Check sheet for the modelled part. Datum: model origin and axes. Units: mm. A direction names the side the tool comes from. Coordinates: 2 decimals unless noted, no trailing zeros. Loops run counter-clockwise (first coordinate to the right, second up) from the corner with the lowest first, then second, coordinate; pieces in that order, holes last. Notation, with made-up numbers: (-21, 3) - (0, 3) arc R8 cw to (0, 13) - close; hole circle Ø11 at (20.5, -30.75). An arc over 180 degrees is marked (long way). Write each question's results on one line, items separated by ' | '. Start each with the question number.
1. Gauge pin test, flat ends, axial feed: P1, Ø4, axis at y = 17, z = -13, coming from the -X side; P2, Ø4, axis at y = -12, z = 7.5, coming from the +X side; P3, Ø12, axis at x = -49.21, y = 4.19, coming from the -Z side; P4, Ø5, axis at y = -0.5, z = 9.5, coming from the +X side. Record the tip position at first contact, or that the pin passes through.
2. Cross-section at B-B (x = 48). Record the cut outline in (y, z), and give its area (3 significant figures).
3. Tool access check on faces 1 (the face through (-66, 3, 12.7)), 2 (the face through (-76.2, 3, 19)), 3 (the face through (-28.1, 12.878, -23.754)), 4 (the face through (-56, 6, 21.158)), 5 (the face through (42.78, 6.22, 23.25)). Record the directions out of +Z, -Z, +X, -X, +Y, -Y that give a thin tool (end or side, any length) a straight path to the whole face; none if there is none.
4. Thickness scan on line 1 (Y direction, x = 16.5, z = -19); line 2 (X direction, y = 8, z = 19.5); line 3 (Y direction, x = -45, z = 14.5). Record the ranges inside material, lowest first. Write a range as [from, to].
5. Cross-section at D-D (x = 13). Record the cut outline in (y, z).
6. Cross-section at C-C (z = 18). Record the cut outline in (x, y), and give its area (3 significant figures).
7. Draft check along Y on faces 6 (the face through (-1, -19.05, 6)), 7 (the face through (39.894, 0.792, 15.794)), 8 (the face through (65, 3, 12.7)). Enter one of: released by +Y, released by -Y, zero draft, split by the parting line, or undercut.
8. Cross-section at A-A (y = 16). Record the cut outline in (x, z).
```python
from build123d import *

# Parameters (mm, degrees)
BOSS_EXTRUDE1_DEPTH     = 25.4
BOSS_EXTRUDE2_DEPTH     = 6.604
SKETCH3_W               = 152.4
SKETCH3_H               = 50.8
BOSS_EXTRUDE3_DEPTH     = 12.446
SKETCH5_W               = 47.049242613
SKETCH5_H               = 38.1
CUT_EXTRUDE1_DEPTH      = 92.800885072
FILLET1_R               = 2.54
FILLET2_R               = 25.4
CUT_EXTRUDE2_DEPTH      = 8.4582
CUT_EXTRUDE2_DEPTH_BACK = 85.242269675
CUT_EXTRUDE2_START      = 12.7
SKETCH6_R               = 9.9187
SKETCH7_R               = 6.7437
CUT_EXTRUDE3_DEPTH      = 93.840002113


with BuildPart() as part:
    # Sketch1 → Boss-Extrude1 (new body)
    with BuildSketch(Plane(origin=(0, 0, 0), x_dir=(1, 0, 0), z_dir=(0, 1, 0))):
        with BuildLine():
            Line((76.2, -25.4), (76.2, 25.4))
            Line((76.2, 25.4), (29.150757387, 25.4))
            ThreePointArc((29.150757387, 25.4), (0, 19.601553837), (-29.150757387, 25.4))
            Line((-29.150757387, 25.4), (-76.2, 25.4))
            Line((-76.2, 25.4), (-76.2, -25.4))
            Line((-76.2, -25.4), (76.2, -25.4))
        make_face()
    extrude(amount=BOSS_EXTRUDE1_DEPTH)

    # Sketch2 → Boss-Extrude2 (add)
    with BuildSketch(Plane.XZ):
        with BuildLine():
            Line((-76.2, 25.4), (76.2, 25.4))
            Line((76.2, 25.4), (76.2, -21.59))
            Line((76.2, -21.59), (29.966893046, -21.59))
            ThreePointArc((29.966893046, -21.59), (0, -15.766153837), (-29.966893046, -21.59))
            Line((-29.966893046, -21.59), (-76.2, -21.59))
            Line((-76.2, -21.59), (-76.2, 25.4))
        make_face()
    extrude(amount=BOSS_EXTRUDE2_DEPTH)

    # Sketch3 → Boss-Extrude3 (add)
    with BuildSketch(Plane.XZ.offset(6.604)):
        Rectangle(SKETCH3_W, SKETCH3_H)
    extrude(amount=BOSS_EXTRUDE3_DEPTH)

    # Sketch5 → Cut-Extrude1 (cut, through all)
    with BuildSketch(Plane(origin=(0, 25.4, 0), x_dir=(1, 0, 0), z_dir=(0, 1, 0))):
        with Locations((-52.675378694, 6.35)):
            Rectangle(SKETCH5_W, SKETCH5_H)
        with Locations((52.675378694, 6.35)):
            Rectangle(SKETCH5_W, SKETCH5_H)
    extrude(amount=-CUT_EXTRUDE1_DEPTH, mode=Mode.SUBTRACT)

    # Fillet1
    fillet1_edges = [part.edges().sort_by_distance(p)[0] for p in [
        (29.150757387, 12.7, -25.4),
        (-29.150757387, 12.7, -25.4),
        (-29.150757387, -12.827, -25.4),
        (-29.150757387, -3.302, -21.265527456),
        (29.150757387, -12.827, -25.4),
        (29.150757387, -3.302, -21.265527456),
    ]]
    fillet(fillet1_edges, radius=FILLET1_R)

    # Fillet2
    fillet2_edges = [part.edges().sort_by_distance(p)[0] for p in [
        (-29.150757387, 3.175, 12.7),
        (29.150757387, 3.175, 12.7),
    ]]
    fillet(fillet2_edges, radius=FILLET2_R)

    # Sketch6 → Cut-Extrude2 (cut, two sides: drawn at the far end of the back side and taken through both)
    with BuildSketch(Plane.XY.offset(CUT_EXTRUDE2_START - CUT_EXTRUDE2_DEPTH_BACK)):
        with Locations(Location((49.2125, 4.191, 0), (0, 0, 302.561278337))):
            Circle(SKETCH6_R)
        with Locations(Location((-49.2125, 4.191, 0), (0, 0, 237.438721663))):
            Circle(SKETCH6_R)
    extrude(amount=CUT_EXTRUDE2_DEPTH + CUT_EXTRUDE2_DEPTH_BACK, mode=Mode.SUBTRACT)

    # Sketch7 → Cut-Extrude3 (cut, through all)
    with BuildSketch(Plane(origin=(0, 0, 21.1582), x_dir=(-1, 0, 0), z_dir=(0, 0, -1))):
        with Locations((-49.2125, 4.191)):
            Circle(SKETCH7_R)
        with Locations((49.2125, 4.191)):
            Circle(SKETCH7_R)
    extrude(amount=-CUT_EXTRUDE3_DEPTH, mode=Mode.SUBTRACT)


solid = part.part
```
Established:
1) P1: x = -29.21 | P2: x = 42.21 | P3: through | P4: x = 42.38
2) outline: (-19.05, 11.84) - (-5.65, 11.84) - (-5.65, 21.16) - (-2.44, 21.16) - (-2.44, 25.4) - (-19.05, 25.4) - close; (10.82, 21.16) - (14.04, 21.16) - (14.04, 11.84) - (25.4, 11.84) - (25.4, 25.4) - (10.82, 25.4) - close | area: 363 mm^2
3) face 1: -Z, -X, +Y, -Y | face 2: +Z, -Z, -X, +Y, -Y | face 3: -Z, +Y | face 4: -Z | face 5: +Z, -Z
4) line 1: [-19.05, -6.6], [0, 25.4] | line 2: [-76.2, -58.37], [-40.05, 40.05], [58.37, 76.2] | line 3: [-19.05, -4.79], [13.17, 25.4]
5) outline: (-19.05, -25.4) - (-6.6, -25.4) - (-6.6, -16.83) - (0, -16.83) - (0, -20.72) - (25.4, -20.72) - (25.4, 25.4) - (-19.05, 25.4) - close
6) outline: (-76.2, -19.05) - (76.2, -19.05) - (76.2, 25.4) - (-76.2, 25.4) - close; hole circle Ø19.84 at (-49.21, 4.19); hole circle Ø19.84 at (49.21, 4.19) | area: 6,160 mm^2
7) face 6: released by -Y | face 7: undercut | face 8: zero draft
8) outline: (-76.2, 12.7) - (-54.55, 12.7) arc R25.4 cw to (-29.15, -12.7) - (-29.15, -21.7) arc R2.54 ccw to (-25.75, -24.09) arc R76.17 cw to (25.75, -24.09) arc R2.54 ccw to (29.15, -21.7) - (29.15, -12.7) arc R25.4 cw to (54.55, 12.7) - (76.2, 12.7) - (76.2, 25.4) - (-76.2, 25.4) - close
